from build123d import *

# Parameters (mm, degrees)
F0_R     = 85.725
F0_R_2   = 1.8288
F0_R_3   = 79.375
F1_DEPTH = 3.175


with BuildPart() as f1:
    # F0 (on Top) → F1 (new body)
    with BuildSketch(Plane.XY):
        Circle(F0_R)
        with Locations((-41.275, -71.490397)):
            Circle(F0_R_2, mode=Mode.SUBTRACT)
        with Locations((0, -82.55)):
            Circle(F0_R_2, mode=Mode.SUBTRACT)
        with Locations((41.275, -71.490397)):
            Circle(F0_R_2, mode=Mode.SUBTRACT)
        with Locations((-82.55, 0)):
            Circle(F0_R_2, mode=Mode.SUBTRACT)
        with Locations((-71.490397, 41.275)):
            Circle(F0_R_2, mode=Mode.SUBTRACT)
        with Locations((-41.275, 71.490397)):
            Circle(F0_R_2, mode=Mode.SUBTRACT)
        Circle(F0_R_3, mode=Mode.SUBTRACT)
        with Locations((82.55, 0)):
            Circle(F0_R_2, mode=Mode.SUBTRACT)
        with Locations((71.490397, 41.275)):
            Circle(F0_R_2, mode=Mode.SUBTRACT)
        with Locations((41.275, 71.490397)):
            Circle(F0_R_2, mode=Mode.SUBTRACT)
    extrude(amount=F1_DEPTH)


solid = f1.part
Read the model definition and answer for the solid it produces. Units are mm, in the model's axes. Round coordinates to 2 decimals unless told otherwise and drop trailing zeros. Write each loop counter-clockwise with the first axis right and the second up, starting at its lowest first coordinate (ties: lowest second). Pieces come first, ordered by that corner, then holes.
Q1. Straight lines are drawn through the part: line 1 (Y direction, x = 0, z = 1.05) (3 decimals); line 2 (X direction, y = 72, z = 1.25); line 3 (X direction, y = -18, z = 2). For each, find the intervals that lie inside material, in ascending order.
Values:
line 1: y = -85.725 to -84.379, -80.721 to -79.375, 79.375 to 85.725
line 2: x = -46.53 to -43.03, -39.52 to -33.41, 33.41 to 39.52, 43.03 to 46.53
line 3: x = -83.81 to -77.31, 77.31 to 83.81
Q2. Find section B-B on x = -67. Determine the outline of the cut face in (y, z) (3 decimals).
Values:
outline: (-53.477, 0) - (-42.56, 0) - (-42.56, 3.175) - (-53.477, 3.175) - close; (42.56, 0) - (53.477, 0) - (53.477, 3.175) - (42.56, 3.175) - close
Q3. Flat-ended cylindrical pins translate along their axes: P1, Ø1, axis at y = 3.5, z = 1, coming from the +X side; P2, Ø1, axis at x = 67, z = 1.5, coming from the +Y side. Find the tip coordinate at first contact, or state that the pin passes through.
Values:
P1: stops at x = 85.67
P2: stops at y = 54.1
Q4. Find section A-A on y = 33.5. Determine the outline of the cut face in (x, z) (3 decimals), and give its area (3 significant figures).
Values:
outline: (-78.908, 0) - (-71.959, 0) - (-71.959, 3.175) - (-78.908, 3.175) - close; (71.959, 0) - (78.908, 0) - (78.908, 3.175) - (71.959, 3.175) - close
area: 44.1 mm2
Q5. The mould has two halves that part along Y. Classify faces 1 (the face through (-69.746, 41.824, 1.565)), 2 (the face through (46.09, 72.28, 1.57)), 3 (the face through (76, -25, 3.175)): released by +Y, released by -Y, zero draft, split by the parting line, or undercut.
Values:
face 1: undercut
face 2: split by the parting line
face 3: zero draft
Q6. Find section C-C on z = 2.15. State how many separate pieces and enclosed holes the cut face has, and give its area (3 significant figures).
Values:
separate pieces: 1
enclosed holes: 10
area: 3,200 mm2
